Could you check a few things on this model? Use its own coordinates, in mm. Round coordinates to 2 decimals unless told otherwise and drop trailing zeros. Order: outer loops, then holes, each group sorted by start corner. A loop starts at its lowest first (then second) coordinate and runs counter-clockwise, first axis right, second up.
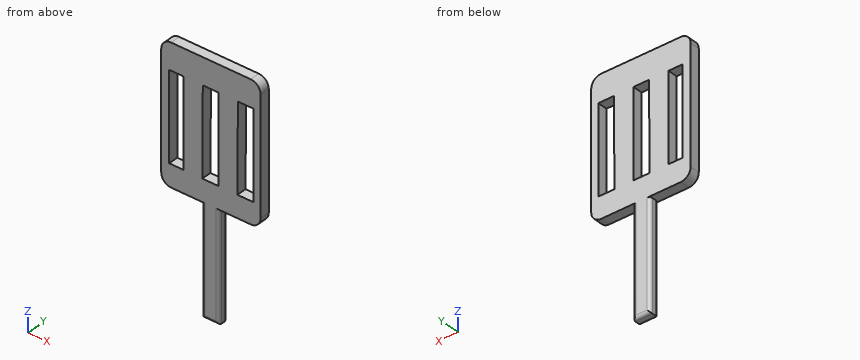
```python
from build123d import *

# Parameters (mm, degrees)
F0_W     = 8.723831
F0_H     = 55.245
F1_DEPTH = 5.08
F2_R     = 5.08
F3_R     = 5.08
F4_R     = 1.5875


with BuildPart() as f1:
    # F0 (on Front) → F1 (new body)
    with BuildSketch(Plane.XZ):
        Polygon((-25.729871, 69.29215), (-25.729871, 0), (-4.985048, 0), (3.738783, 0), (25.070129, 0), (25.070129, 69.29215), align=None)
        Polygon((-21.684954, 11.216355), (-21.684954, 51.844489), (-21.684954, 55.832524), (-14.456635, 55.832524), (-14.456635, 11.216355), align=None, mode=Mode.SUBTRACT)
        Polygon((-4.735794, 11.216355), (-4.486542, 55.832524), (3.489533, 55.832524), (3.489533, 11.216355), align=None, mode=Mode.SUBTRACT)
        Polygon((13.210376, 11.216355), (13.459626, 55.832524), (21.4357, 55.832524), (21.4357, 11.216355), align=None, mode=Mode.SUBTRACT)
        with Locations((-0.623133, -27.6225)):
            Rectangle(F0_W, F0_H)
    extrude(amount=F1_DEPTH)

    # F2
    f2_edges = [f1.edges().sort_by_distance(p)[0] for p in [
        (-25.729871, -2.54, 69.29215),
        (25.070129, -2.54, 69.29215),
    ]]
    fillet(f2_edges, radius=F2_R)

    # F3
    f3_edges = [f1.edges().sort_by_distance(p)[0] for p in [
        (-25.729871, -2.54, 0),
        (25.070129, -2.54, 0),
    ]]
    fillet(f3_edges, radius=F3_R)

    # F4
    f4_edges = [f1.edges().sort_by_distance(p)[0] for p in [
        (3.738783, 0, -27.6225),
        (-0.623132, 0, -55.245),
        (-4.985048, 0, -27.6225),
        (3.738783, -5.08, -27.6225),
        (-4.985048, -5.08, -27.6225),
        (-0.623132, -5.08, -55.245),
    ]]
    fillet(f4_edges, radius=F4_R)


solid = f1.part
```
Q1. I need wall thicknesses on L1, parallel to Z at x = -17, y = -4.5; L2, parallel to X at y = -2.5, z = 12; L3, parallel to X at y = -4.5, z = 49.5. Which ranges of each line are inside material? Lowest first, please.
Q2. For P1, Ø0.6, axis at y = -2.5, z = -31, coming from the -X side; P2, Ø2.5, axis at x = -14.5, y = -3.5, coming from the -Z side; P3, Ø1.5, axis at y = -2.5, z = -40.5, coming from the +X side, each with a flat end and sliding along its axis, tell me the tip position at first contact or that it passes through.
Q3. Imagine slicing it at C-C, the plane z = -9. Please give me the cut outline in (x, y) (1 decimal).
Q4. Imagine slicing it at B-B, the plane z = 17. Please give me the cut outline in (x, y), then the cut area to 3 significant figures.
Q5. Imagine slicing it at D-D, the plane x = 6.5. Please give me the cut outline in (y, z).
Q6. Imagine slicing it at A-A, the plane x = -2. Please give me the cut outline in (y, z) (1 decimal).
Filled in:
1. L1: z = 0 to 11.22, 55.83 to 69.29
1. L2: x = -25.73 to -21.68, -14.46 to -4.73, 3.49 to 13.21, 21.44 to 25.07
1. L3: x = -25.73 to -21.68, -14.46 to -4.52, 3.49 to 13.42, 21.44 to 25.07
2. P1: stops at x = -4.99
2. P2: stops at z = 0
2. P3: stops at x = 3.74
3. outline: (-5, -3.5) arc R1.6 ccw to (-3.4, -5.1) - (2.2, -5.1) arc R1.6 ccw to (3.7, -3.5) - (3.7, -1.6) arc R1.6 ccw to (2.2, 0) - (-3.4, 0) arc R1.6 ccw to (-5, -1.6) - close
4. outline: (-25.73, -5.08) - (-21.68, -5.08) - (-21.68, 0) - (-25.73, 0) - close; (-14.46, -5.08) - (-4.7, -5.08) - (-4.7, 0) - (-14.46, 0) - close; (3.49, -5.08) - (13.24, -5.08) - (13.24, 0) - (3.49, 0) - close; (21.44, -5.08) - (25.07, -5.08) - (25.07, 0) - (21.44, 0) - close
4. area: 138 mm2
5. outline: (-5.08, 0) - (0, 0) - (0, 69.29) - (-5.08, 69.29) - close
6. outline: (-5.1, -53.7) arc R1.6 ccw to (-3.5, -55.2) - (-1.6, -55.2) arc R1.6 ccw to (0, -53.7) - (0, 11.2) - (-5.1, 11.2) - close; (-5.1, 55.8) - (0, 55.8) - (0, 69.3) - (-5.1, 69.3) - close
